Design review of the part built by this model. Coordinates are the model's own, in mm. Give positions to 0.01 mm unless a question says otherwise; leave off trailing zeros. Write each loop counter-clockwise with the first axis right and the second up, starting at its lowest first coordinate (ties: lowest second). Pieces come first, ordered by that corner, then holes. Notation, with made-up numbers: (46.5, 35.5) -> (100.5, 35.5) arc R12 ccw to (100.5, 54.5) -> close; hole circle Ø1 at (29.25, 76). An arc over 180 degrees is marked (long way). Use CSV: the item, a comma, the result in double quotes.
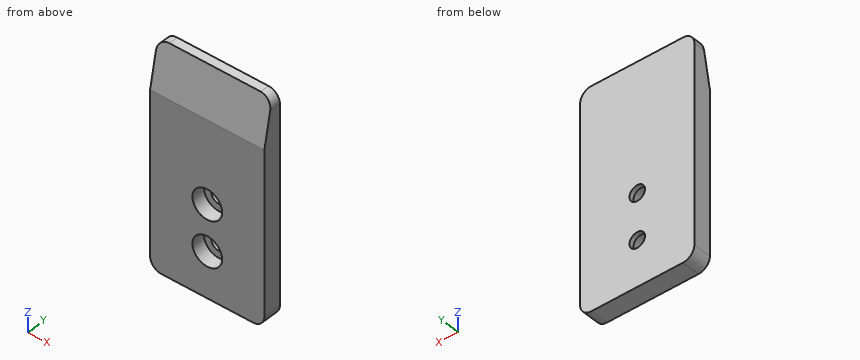
```python
from build123d import *

# Parameters (mm, degrees)
SKETCH1_W                      = 25
SKETCH1_H                      = 30
BOSS_EXTRUDE1_DEPTH            = 4
CBORE_FOR_M3_SHCS2_D           = 3.4
CBORE_FOR_M3_SHCS2_CBORE_D     = 6.5
CBORE_FOR_M3_SHCS2_CBORE_DEPTH = 3
SKETCH5_W                      = 25
SKETCH5_H                      = 4
BOSS_EXTRUDE2_DEPTH            = 18
CHAMFER1_SIZE                  = 10
CHAMFER1_SIZE2                 = 2
FILLET1_R                      = 2.5


with BuildPart() as part:
    # Sketch1 → Boss-Extrude1 (new body)
    with BuildSketch(Plane(origin=(0, 0, 0), x_dir=(1, 0, 0), z_dir=(0, 1, 0))):
        with Locations((12.5, 15)):
            Rectangle(SKETCH1_W, SKETCH1_H)
    extrude(amount=BOSS_EXTRUDE1_DEPTH)

    # CBORE for M3 SHCS2 (through all)
    with Locations(Plane(origin=(0, 0, 0), x_dir=(-1, 0, 0), z_dir=(0, -1, 0))):
        with Locations((-12.5, 20), (-12.5, 10)):
            CounterBoreHole(CBORE_FOR_M3_SHCS2_D / 2, CBORE_FOR_M3_SHCS2_CBORE_D / 2, CBORE_FOR_M3_SHCS2_CBORE_DEPTH)

    # Sketch5 → Boss-Extrude2 (add)
    with BuildSketch(Plane.XY):
        with Locations((12.5, 2)):
            Rectangle(SKETCH5_W, SKETCH5_H)
    extrude(amount=BOSS_EXTRUDE2_DEPTH)

    # Chamfer1
    chamfer1_edges = [part.edges().sort_by_distance(p)[0] for p in [
        (12.5, 0, 18),
    ]]
    chamfer1_side = [part.faces().sort_by_distance(p)[0] for p in [
        (12.5, 0, -5.473114445),
    ]]
    chamfer(chamfer1_edges, length=CHAMFER1_SIZE, length2=CHAMFER1_SIZE2, reference=chamfer1_side[0])

    # Fillet1
    fillet1_edges = [part.edges().sort_by_distance(p)[0] for p in [
        (0, 3, 18),
        (25, 3, 18),
        (0, 2, -30),
        (25, 2, -30),
    ]]
    fillet(fillet1_edges, radius=FILLET1_R)


solid = part.part
```
(1) Take a section at A-A (x = 12.5). Write out the cut boundary in (y, z), then the cut area to 3 significant figures.
Established:
outline,"(0, -30) -> (4, -30) -> (4, -21.7) -> (3, -21.7) -> (3, -23.25) -> (0, -23.25) -> close; (0, -16.75) -> (3, -16.75) -> (3, -18.3) -> (4, -18.3) -> (4, -11.7) -> (3, -11.7) -> (3, -13.25) -> (0, -13.25) -> close; (0, -6.75) -> (3, -6.75) -> (3, -8.3) -> (4, -8.3) -> (4, 18) -> (2, 18) -> (0, 8) -> close"
area,"136 mm2"
(2) Take a section at C-C (y = 3.5). Write out the cut boundary in (x, z).
Established:
outline,"(0, -27.5) arc R2.5 ccw to (2.5, -30) -> (22.5, -30) arc R2.5 ccw to (25, -27.5) -> (25, 15.5) arc R2.5 ccw to (22.5, 18) -> (2.5, 18) arc R2.5 ccw to (0, 15.5) -> close; hole circle Ø3.4 at (12.5, -20); hole circle Ø3.4 at (12.5, -10)"
(3) Take a section at D-D (x = 7.5). Write out the cut boundary in (y, z), then the cut area to 3 significant figures.
Established:
outline,"(0, -30) -> (4, -30) -> (4, 18) -> (2, 18) -> (0, 8) -> close"
area,"182 mm2"
(4) For line 1 along Z through (x, y) = (12.5, 2.35); line 2 along Z through (x, y) = (12.5, 3.4); line 3 along X through (y, z) = (3.6, -10), list the stretches that pass through material, from the lowest coordinate up. Write a range as [from, to].
Established:
line 1,"z = [-30, -23.25], [-16.75, -13.25], [-6.75, 18]"
line 2,"z = [-30, -21.7], [-18.3, -11.7], [-8.3, 18]"
line 3,"x = [0, 10.8], [14.2, 25]"
(5) Clearance check with a flat-ended pin moving along its axis: pin 1 (3 mm diameter, centred on x = 11.5, z = -21, fed in from -Y). State where the tip first meets the part, or that it passes through.
Established:
pin 1,"stops at y = 3"
(6) Take a section at B-B (z = -10). Write out the cut boundary in (x, y), then the cut area to 3 significant figures.
Established:
outline,"(0, 0) -> (9.25, 0) -> (9.25, 3) -> (10.8, 3) -> (10.8, 4) -> (0, 4) -> close; (14.2, 3) -> (15.75, 3) -> (15.75, 0) -> (25, 0) -> (25, 4) -> (14.2, 4) -> close"
area,"77.1 mm2"
